from build123d import *

# Parameters (mm, degrees)
F0_R     = 7.50062
F1_DEPTH = 105.00106
F3_R     = 9.99998
F4_DEPTH = 2.49936
F6_R     = 9.99998
F7_DEPTH = 2.49936
F8_SIZE  = 0.999998


with BuildPart() as f1:
    # F0 (on Front) → F1 (new body)
    with BuildSketch(Plane.XZ):
        Circle(F0_R)
    extrude(amount=-F1_DEPTH)

    # F3 (on offset) → F4 (join)
    with BuildSketch(Plane.XZ.offset(-15.00124)):
        Circle(F3_R)
    extrude(amount=-F4_DEPTH)

    # F6 (on offset) → F7 (join)
    with BuildSketch(Plane(origin=(0, 89.99982, 0), x_dir=(1, 0, 0), z_dir=(0, 1, 0))):
        Circle(F6_R)
    extrude(amount=-F7_DEPTH)

    # F8
    f8_edges = [f1.edges().sort_by_distance(p)[0] for p in [
        (-9.99998, 15.00124, 0),
        (-9.99998, 89.99982, 0),
    ]]
    chamfer(f8_edges, length=F8_SIZE)


solid = f1.part
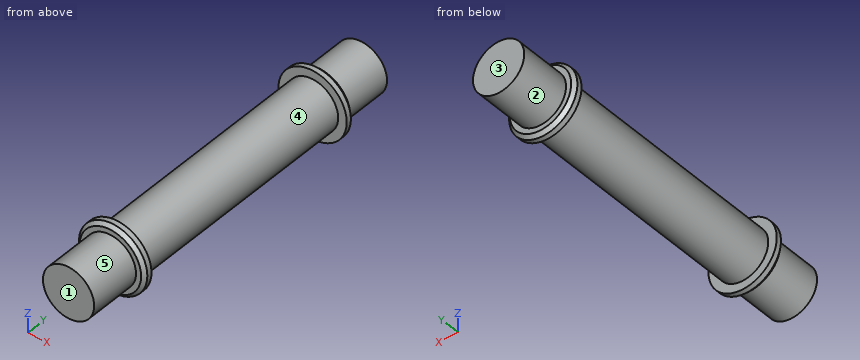
Build history of the part. All positions in model axes, mm. Face numbers are marked on the shaded views. A direction names the side the tool comes from. Round coordinates to 2 decimals unless told otherwise and drop trailing zeros. Write each loop counter-clockwise with the first axis right and the second up, starting at its lowest first coordinate (ties: lowest second). Pieces come first, ordered by that corner, then holes. Notation, with made-up numbers: M -8,69 L 22,69 A34 ccw 22,103 Z; hole C 60.5,17 d4. An arc over 180 degrees is marked long. Answer in a Markdown table with one row per item.
1. Which spindle directions (+Z, -Z, +X, -X, +Y, -Y) get a long thin tool onto all of the face, cutting with end or side? Do the marked faces 1 and 2. Say none if no direction does.
Geometry check:
| item | result |
|---|---|
| face 1 | +Z, -Z, +X, -X, -Y |
| face 2 | +Y |
2. Saw through at B-B (x = 0). List the corners of the cut face in (y, z).
Geometry check:
| item | result |
|---|---|
| outline | M 0,-7.5 L 15,-7.5 L 15,-9 L 16,-10 L 17.5,-10 L 17.5,-7.5 L 87.5,-7.5 L 87.5,-10 L 89,-10 L 90,-9 L 90,-7.5 L 105,-7.5 L 105,7.5 L 90,7.5 L 90,9 L 89,10 L 87.5,10 L 87.5,7.5 L 17.5,7.5 L 17.5,10 L 16,10 L 15,9 L 15,7.5 L 0,7.5 Z |
3. Saw through at C-C (y = 39). List the corners of the cut face in (x, z), and give its area (3 significant figures).
Geometry check:
| item | result |
|---|---|
| outline | C 0,0 d15 |
| area | 177 mm2 |
4. Mould opens along Y. For the marked faces 3, 4 and 5 say: +Y half, -Y half, draft (parallel to the pull), parting line (faces both ways), or undercut.
Geometry check:
| item | result |
|---|---|
| face 3 | +Y half |
| face 4 | undercut |
| face 5 | draft |
5. Saw through at A-A (z = 0). List the corners of the cut face in (x, y), and give its area (3 significant figures).
Geometry check:
| item | result |
|---|---|
| outline | M -10,16 L -9,15 L -7.5,15 L -7.5,0 L 7.5,0 L 7.5,15 L 9,15 L 10,16 L 10,17.5 L 7.5,17.5 L 7.5,87.5 L 10,87.5 L 10,89 L 9,90 L 7.5,90 L 7.5,105 L -7.5,105 L -7.5,90 L -9,90 L -10,89 L -10,87.5 L -7.5,87.5 L -7.5,17.5 L -10,17.5 Z |
| area | 1,600 mm2 |
6. Probe L1, parallel to Y at x = -5.5, z = 6.5; L2, parallel to Y at x = -6, z = 7.25; L3, parallel to Z at x = -6.25, y = 25.5. List the from-to ranges inside material, lowest first. Write a range as [from, to].
Geometry check:
| item | result |
|---|---|
| L1 | [15, 17.5], [87.5, 90] |
| L2 | [15.41, 17.5], [87.5, 89.59] |
| L3 | [-4.15, 4.15] |
7. Flat gauge pins, fed straight in: P1, Ø5, axis at y = 22, z = -1.5, coming from the +X side; P2, Ø5, axis at y = 56.5, z = -3.5, coming from the +X side; P3, Ø4, axis at x = -7.5, y = 14.5, coming from the -Z side. Where does each tip first touch, or does it go through?
Geometry check:
| item | result |
|---|---|
| P1 | x = 7.5 |
| P2 | x = 7.43 |
| P3 | z = -7.86 |
